```python
from build123d import *

# Parameters (mm, degrees)
SCHIZZO1_R                   = 60
SCHIZZO1_R_2                 = 48
ESTRUSIONE_ESTRUSIONE1_DEPTH = 5
RIVOLUZIONE1_ANGLE           = 23
RIVOLUZIONE1_OTHER_WAY_ANGLE = 23
RIVOLUZIONE2_ANGLE           = 3
RIVOLUZIONE3_ANGLE           = 3


with BuildPart() as part:
    # Schizzo1 → Estrusione-Estrusione1 (new body)
    with BuildSketch(Plane(origin=(0, 0, 0), x_dir=(1, 0, 0), z_dir=(0, 1, 0))):
        with Locations(Location((0, 0, 0), (0, 0, 270))):
            Circle(SCHIZZO1_R)
        with Locations(Location((0, 0, 0), (0, 0, 270))):
            Circle(SCHIZZO1_R_2, mode=Mode.SUBTRACT)
        with BuildLine():
            ThreePointArc((-14.558571287, -54.333327729), (0, -56.25), (14.558571287, -54.333327729))
            ThreePointArc((14.558571287, -54.333327729), (16.149561545, -51.577651768), (13.393885584, -49.98666151))
            ThreePointArc((13.393885584, -49.98666151), (0, -51.75), (-13.393885584, -49.98666151))
            ThreePointArc((-13.393885584, -49.98666151), (-16.149561545, -51.577651768), (-14.558571287, -54.333327729))
        make_face(mode=Mode.SUBTRACT)
        with BuildLine():
            ThreePointArc((13.393885584, 49.98666151), (16.149561545, 51.577651768), (14.558571287, 54.333327729))
            ThreePointArc((14.558571287, 54.333327729), (0, 56.25), (-14.558571287, 54.333327729))
            ThreePointArc((-14.558571287, 54.333327729), (-16.149561545, 51.577651768), (-13.393885584, 49.98666151))
            ThreePointArc((-13.393885584, 49.98666151), (0, 51.75), (13.393885584, 49.98666151))
        make_face(mode=Mode.SUBTRACT)
        with BuildLine():
            ThreePointArc((49.98666151, -13.393885584), (51.577651768, -16.149561545), (54.333327729, -14.558571287))
            ThreePointArc((54.333327729, -14.558571287), (56.25, 0), (54.333327729, 14.558571287))
            ThreePointArc((54.333327729, 14.558571287), (51.577651768, 16.149561545), (49.98666151, 13.393885584))
            ThreePointArc((49.98666151, 13.393885584), (51.75, 0), (49.98666151, -13.393885584))
        make_face(mode=Mode.SUBTRACT)
        with BuildLine():
            ThreePointArc((-49.98666151, 13.393885584), (-51.577651768, 16.149561545), (-54.333327729, 14.558571287))
            ThreePointArc((-54.333327729, 14.558571287), (-56.25, 0), (-54.333327729, -14.558571287))
            ThreePointArc((-54.333327729, -14.558571287), (-51.577651768, -16.149561545), (-49.98666151, -13.393885584))
            ThreePointArc((-49.98666151, -13.393885584), (-51.75, 0), (-49.98666151, 13.393885584))
        make_face(mode=Mode.SUBTRACT)
    extrude(amount=ESTRUSIONE_ESTRUSIONE1_DEPTH)

    # Schizzo2 → Rivoluzione1 (revolve)
    with BuildSketch(Plane.ZY):
        Polygon((83.801322108, 10.249602265), (156.30594507, -23.559858674), (154.630778704, -17.261826174), (64, 25), (60, 25), (60, 0), (72, 0), (75.34408852, 7.171420975), align=None)
    revolve(axis=Axis((0, 115.29923816, 0), (0, -1, 0)), revolution_arc=RIVOLUZIONE1_ANGLE)

    # Schizzo2 → Rivoluzione1 other way (revolve)
    with BuildSketch(Plane.ZY):
        Polygon((83.801322108, 10.249602265), (156.30594507, -23.559858674), (154.630778704, -17.261826174), (64, 25), (60, 25), (60, 0), (72, 0), (75.34408852, 7.171420975), align=None)
    revolve(axis=Axis((0, 115.29923816, 0), (0, 1, 0)), revolution_arc=RIVOLUZIONE1_OTHER_WAY_ANGLE)

    # Schizzo3 → Rivoluzione2 (revolve)
    with BuildSketch(Plane(origin=(0, 0, 0), x_dir=(-0.39073112848927466, 0, 0.92050485345244), z_dir=(-0.92050485345244, 0, -0.39073112848927466))):
        Polygon((60, 25), (60, 30), (64, 30), (156.743870012, -12.730287239), (154.630778704, -17.261826174), (64, 25), align=None)
    revolve(axis=Axis((0, 115.29923816, 0), (0, 1, 0)), revolution_arc=RIVOLUZIONE2_ANGLE)

    # Schizzo4 → Rivoluzione3 (revolve)
    with BuildSketch(Plane(origin=(0, 0, 0), x_dir=(-0.39073112848927455, 0, -0.92050485345244), z_dir=(0.92050485345244, 0, -0.39073112848927455))):
        Polygon((-60, 25), (-64, 25), (-154.630778704, -17.261826174), (-154.630778704, -12.261826174), (-64, 30), (-60, 30), align=None)
    revolve(axis=Axis((0, 115.29923816, 0), (0, -1, 0)), revolution_arc=RIVOLUZIONE3_ANGLE)


solid = part.part
```
Here's how the part is built. I have some questions about the finished solid (model axes, mm). A direction names the side the tool comes from. Coordinates: 2 decimals unless noted, no trailing zeros. Write each loop counter-clockwise with the first axis right and the second up, starting at its lowest first coordinate (ties: lowest second). Pieces come first, ordered by that corner, then holes. Notation, with made-up numbers: (37, -37.75) -> (55, -37.75) arc R24 ccw to (55, -24.75) -> close; hole circle Ø3 at (8.5, -14). An arc over 180 degrees is marked (long way). Use a Markdown table: item, result. Add a question column.
(1) We'd pull the mould along X, two halves only. Please class faces 3 (the cylindrical face through (-51.626, 2.465, 16.162)), 4 (the flat face through (-23, 30, 58)), 5 (the conical face through (-0.87, -19.67, 155.27)): +X half, -X half, draft (parallel to the pull), parting line (faces both ways), or undercut.
(2) I'm going to push flat-ended pins straight in: P1, Ø8.5, axis at x = 3.5, z = 61.5, coming from the +Y side; P2, Ø2, axis at x = 38.5, y = 12, coming from the +Z side; P3, Ø2, axis at x = 2, y = 21, coming from the -Z side. Where does each tip first touch, or does it pass through?
(3) If we section it at C-C, the plane z = 43: Write out the boundary of the cut face in (x, y).
(4) If we section it at A-A, the plane z = 0: Write out the boundary of the cut face in (x, y).
(5) If we section it at D-D, the plane y = -9.5: Write out the boundary of the cut face in (x, z), and give its area (3 significant figures).
(6) For faces 1 (the cylindrical face through (51.75, 2.46, -0.19)), 2 (the flat face through (-37.143, 6.479, 102.048)), which set-ups out of +Z, -Z, +X, -X, +Y, -Y let a thin tool reach every point of the face, with its end or its side?
(7) If we section it at B-B, the plane x = 0: Write out the boundary of the cut face in (y, z), and give its area (3 significant figures).
(8) Please list where these lines run through material, in increasing order: line 1 (Y direction, x = -17.5, z = -46); line 2 (Z direction, x = -33, y = 0.5); line 3 (X direction, y = 2, z = -21).
Outcome:
| question | item | result |
|---|---|---|
| 1 | face 3 | undercut |
| 1 | face 4 | draft |
| 1 | face 5 | parting line |
| 2 | P1 | stops at y = 25 |
| 2 | P2 | stops at z = 97.45 |
| 2 | P3 | stops at z = 59.92 |
| 3 | outline | (-41.84, 0) -> (-21.33, 0) -> (-21.33, 5) -> (-41.84, 5) -> close; (21.33, 0) -> (41.84, 0) -> (41.84, 5) -> (21.33, 5) -> close |
| 4 | outline | (-60, 0) -> (-56.25, 0) -> (-56.25, 5) -> (-60, 5) -> close; (-51.75, 0) -> (-48, 0) -> (-48, 5) -> (-51.75, 5) -> close; (48, 0) -> (51.75, 0) -> (51.75, 5) -> (48, 5) -> close; (56.25, 0) -> (60, 0) -> (60, 5) -> (56.25, 5) -> close |
| 5 | outline | (-58.51, 137.83) -> (-49.29, 116.13) arc R126.15 cw to (49.29, 116.13) -> (58.1, 136.89) arc R148.71 ccw to (50.86, 139.74) -> (47.19, 129.66) arc R137.99 ccw to (-47.19, 129.66) -> (-51.21, 140.7) arc R149.73 ccw to start |
| 5 | area | 1,420 mm^2 |
| 6 | face 1 | +Y, -Y |
| 6 | face 2 | +Z, +Y |
| 7 | outline | (-23.56, 156.31) -> (10.25, 83.8) -> (7.17, 75.34) -> (0, 72) -> (0, 56.25) -> (5, 56.25) -> (5, 60) -> (25, 60) -> (25, 64) -> (-17.26, 154.63) -> close; (0, -60) -> (5, -60) -> (5, -56.25) -> (0, -56.25) -> close; (0, -51.75) -> (5, -51.75) -> (5, -48) -> (0, -48) -> close; (0, 48) -> (5, 48) -> (5, 51.75) -> (0, 51.75) -> close |
| 7 | area | 888 mm^2 |
| 8 | line 1 | y = 0 to 5 |
| 8 | line 2 | z = -50.11 to -34.86, 34.86 to 50.11, 99.37 to 111.77 |
| 8 | line 3 | x = -56.2 to -43.16, 43.16 to 56.2 |
